Read the model definition and answer for the solid it produces. Units are mm, in the model's axes. A direction names the side the tool comes from. Round coordinates to 2 decimals unless told otherwise and drop trailing zeros. Write each loop counter-clockwise with the first axis right and the second up, starting at its lowest first coordinate (ties: lowest second). Pieces come first, ordered by that corner, then holes. Notation, with made-up numbers: M 34,10 L 65,10 A26 ccw 65,25 Z; hole C -30.75,-20.75 d3. An arc over 180 degrees is marked long. Use one line per item in the form item = value. Start each with the question number.
```python
from build123d import *

# Parameters (mm, degrees)
EXTRUDE_4_DEPTH     = 9.5
SKETCH_11_R         = 2.1
CUT_EXTRUDE_8_DEPTH = 187.923112536
SKETCH_12_R         = 4
CUT_EXTRUDE_9_DEPTH = 1
FILLET_7_R          = 3


with BuildPart() as part:
    # 草图10 → 凸台-拉伸4 (new body)
    with BuildSketch(Plane.XY):
        Polygon((0, 0), (65, 0), (65, 175), (21, 175), (21, 127), (0, 35), align=None)
    extrude(amount=EXTRUDE_4_DEPTH)

    # 草图11 → 切除-拉伸8 (cut, through all)
    with BuildSketch(Plane.XY.offset(9.5)):
        with Locations((48, 165)):
            Circle(SKETCH_11_R)
        with Locations((48, 111)):
            Circle(SKETCH_11_R)
    extrude(amount=-CUT_EXTRUDE_8_DEPTH, mode=Mode.SUBTRACT)

    # 草图12 → 切除-拉伸9 (cut)
    with BuildSketch(Plane.XY.offset(9.5)):
        with Locations((48, 165)):
            Circle(SKETCH_12_R)
        with Locations((48, 111)):
            Circle(SKETCH_12_R)
    extrude(amount=-CUT_EXTRUDE_9_DEPTH, mode=Mode.SUBTRACT)

    # 圆角7
    fillet_7_edges = [part.edges().sort_by_distance(p)[0] for p in [
        (21, 175, 4.75),
        (65, 0, 4.75),
        (21, 127, 4.75),
    ]]
    fillet(fillet_7_edges, radius=FILLET_7_R)


solid = part.part
```
Q1. Find section D-D on y = 111. Write down the section's boundary in (x, z).
Q2. For a pull along X with two mould halves and no side action, classify faces 1 (the face through (0, 18, 5)), 2 (the face through (64.1, 0.86, 4.82)), 3 (the face through (45, 175, 5)), 4 (the face through (49.13, 166.77, 4.31)) as +X half, -X half, draft (parallel to the pull), parting line (faces both ways), or undercut.
Q3. Straight lines are drawn through the part: line 1 (Y direction, x = 48, z = 8.95); line 2 (Y direction, x = 48, z = 6.25); line 3 (X direction, y = 165, z = 5). For each, find the intervals that lie inside material, in ascending order. Write a range as [from, to].
Q4. Find section A-A on y = 165. Write down the section's boundary in (x, z).
Q5. Each of these flat-tipped pins is pushed along its axis until it touches: pin 1 Ø6.5 at (x, y) = (47, 111) entering from +Z; pin 2 Ø4 at (x, z) = (21.5, 1.5) entering from +Y; pin 3 Ø3 at (y, z) = (158, 6) entering from -X; pin 4 Ø5 at (x, y) = (48, 165) entering from +Z. Where does it stop, or does it pass through?
Q6. Find section B-B on x = 48. Write down the section's boundary in (y, z), and give its area (3 significant figures).
Q7. Find section C-C on z = 3.75. Write down the section's boundary in (x, y).
Q8. A tool of negligible diameter and unlimited length cuts with its end or side. For faces 5 (the face through (65, 88, 5)), 6 (the face through (21, 150, 5)), 7 (the face through (47.479, 114.966, 9.007)), from which of +Z, -Z, +X, -X, +Y, -Y can it reach the whole face along a straight path? Write none if from no direction.
Response:
q1.outline = M 17.35,0 L 45.9,0 L 45.9,8.5 L 44,8.5 L 44,9.5 L 17.35,9.5 Z; M 50.1,0 L 65,0 L 65,9.5 L 52,9.5 L 52,8.5 L 50.1,8.5 Z
q2.face_1 = -X half
q2.face_2 = +X half
q2.face_3 = draft
q2.face_4 = undercut
q3.line_1 = [0, 107], [115, 161], [169, 175]
q3.line_2 = [0, 108.9], [113.1, 162.9], [167.1, 175]
q3.line_3 = [21, 45.9], [50.1, 65]
q4.outline = M 21,0 L 45.9,0 L 45.9,8.5 L 44,8.5 L 44,9.5 L 21,9.5 Z; M 50.1,0 L 65,0 L 65,9.5 L 52,9.5 L 52,8.5 L 50.1,8.5 Z
q5.pin_1 = 9.5
q5.pin_2 = 174.96
q5.pin_3 = 21
q5.pin_4 = 8.5
q6.outline = M 0,0 L 108.9,0 L 108.9,8.5 L 107,8.5 L 107,9.5 L 0,9.5 Z; M 113.1,0 L 162.9,0 L 162.9,8.5 L 161,8.5 L 161,9.5 L 115,9.5 L 115,8.5 L 113.1,8.5 Z; M 167.1,0 L 175,0 L 175,9.5 L 169,9.5 L 169,8.5 L 167.1,8.5 Z
q6.area = 1,580 mm²
q7.outline = M 0,0 L 62,0 A3 ccw 65,3 L 65,175 L 24,175 A3 ccw 21,172 L 21,127.34 A3 cw 20.92,126.67 L 0,35 Z; hole C 48,111 d4.2; hole C 48,165 d4.2
q8.face_5 = +Z, -Z, +X, +Y, -Y
q8.face_6 = +Z, -Z, -X, +Y
q8.face_7 = +Z
